Here's how the part is built. I have some questions about the finished solid (model axes, mm). A direction names the side the tool comes from. Coordinates: 2 decimals unless noted, no trailing zeros. Write each loop counter-clockwise with the first axis right and the second up, starting at its lowest first coordinate (ties: lowest second). Pieces come first, ordered by that corner, then holes. Notation, with made-up numbers: (-14, 13) -> (22, 13) arc R33 ccw to (22, 41) -> close; hole circle Ø2 at (68, -35). An arc over 180 degrees is marked (long way). Use a Markdown table: item, result. Add a question column.
Item 1: If I drill on line 1 along Y through (x, z) = (0, -0.5); line 2 along Y through (x, z) = (0, 1.5); line 3 along X through (y, z) = (17.5, -0.5), over which ranges is the centre line in solid material (lowest first)? Write a range as from..to.
Item 2: On a 3-axis mill with a long thin cutter (end or side, diameter ignored), from which of +Z, -Z, +X, -X, +Y, -Y can I reach the whole of each face in a straight line? I mean faces 1 (the cylindrical face through (61.522, 19.374, 0.986)), 2 (the flat face through (22.5, 1, -7)), 3 (the cylindrical face through (-62.44, 2.75, 6.44)), 4 (the flat face through (0, -37.5, -4)), 5 (the flat face through (-22.5, 1, -7)). Say none if no direction works.
Item 3: If we mould it in two halves opening along Y, with no side actions, what happens to faces 6 (the flat face through (0, 37.5, -4)), 7 (the cylindrical face through (-0.54, 19.94, 2.83)), 8 (the flat face through (-34, 53, 2))? For each: pulls with the +Y half, pulls with the -Y half, needs draft (parallel to the pull), parting line crosses it, or undercut.
Item 4: Will these pins go through, and if not, where does the flat tip stop? pin 1 Ø4 at (y, z) = (-29, -4.5) entering from -X; pin 2 Ø8 at (x, y) = (0, 17.5) entering from -Z; pin 3 Ø4.5 at (x, z) = (0, -5.5) entering from -Y.
Item 5: Imagine slicing it at C-C, the plane z = -12. Write out the boundary of the cut face in (x, y), and give its area (3 significant figures).
Item 6: Imagine slicing it at A-A, the plane x = 0. Write out the boundary of the cut face in (y, z).
Item 7: Imagine slicing it at B-B, the plane y = -17.5. Write out the boundary of the cut face in (x, z), and give its area (3 significant figures).
Item 8: Imagine slicing it at D-D, the plane x = -19.5. Write out the boundary of the cut face in (y, z), and give its area (3 significant figures).
```python
from build123d import *

# Parameters (mm, degrees)
F0_R      = 64.5
F1_DEPTH  = 2
F2_R      = 62.5
F3_DEPTH  = 9
F4_W      = 45
F4_H      = 75
F5_DEPTH  = 15
F8_DEPTH  = 75
F9_R      = 2.5
F10_DEPTH = 35


with BuildPart() as f1:
    # F0 (on Top) → F1 (new body)
    with BuildSketch(Plane.XY):
        Circle(F0_R)
    extrude(amount=F1_DEPTH)

    # F2 (on face) → F3 (join)
    with BuildSketch(Plane.XY.offset(2)):
        Circle(F2_R)
    extrude(amount=F3_DEPTH)

    # F4 (on face) → F5 (join)
    with BuildSketch(Plane(origin=(0, 0, 0), x_dir=(1, 0, 0), z_dir=(0, 0, -1))):
        Rectangle(F4_W, F4_H)
    extrude(amount=F5_DEPTH)

    # F7 (on face) → F8 (cut)
    with BuildSketch(Plane.XZ.offset(37.5)):
        with BuildLine():
            Line((-22.360679775, -15), (22.360679775, -15))
            ThreePointArc((22.360679775, -15), (0, -5), (-22.360679775, -15))
        make_face()
    extrude(amount=-F8_DEPTH, mode=Mode.SUBTRACT)

    # F9 (on face) → F10 (cut)
    with BuildSketch(Plane(origin=(0, 0, -15), x_dir=(1, 0, 0), z_dir=(0, 0, -1))):
        with Locations((0, 17.5)):
            Circle(F9_R)
        with Locations((0, -17.5)):
            Circle(F9_R)
    extrude(amount=-F10_DEPTH, mode=Mode.SUBTRACT)


solid = f1.part
```
Ans:
| question | item | result |
|---|---|---|
| 1 | line 1 | y = -37.5..-20, -15..15, 20..37.5 |
| 1 | line 2 | y = -64.5..-20, -15..15, 20..64.5 |
| 1 | line 3 | x = -22.5..-2.5, 2.5..22.5 |
| 2 | face 1 | +Z, -Z |
| 2 | face 2 | -Z, +X, +Y, -Y |
| 2 | face 3 | +Z |
| 2 | face 4 | -Z, +X, -X, -Y |
| 2 | face 5 | -Z, -X, +Y, -Y |
| 3 | face 6 | pulls with the +Y half |
| 3 | face 7 | undercut |
| 3 | face 8 | needs draft |
| 4 | pin 1 | stops at x = -22.5 |
| 4 | pin 2 | stops at z = -5.27 |
| 4 | pin 3 | stops at y = -37.5 |
| 5 | outline | (-22.5, -37.5) -> (-19.26, -37.5) -> (-19.26, 37.5) -> (-22.5, 37.5) -> close; (19.26, -37.5) -> (22.5, -37.5) -> (22.5, 37.5) -> (19.26, 37.5) -> close |
| 5 | area | 486 mm^2 |
| 6 | outline | (-64.5, 0) -> (-37.5, 0) -> (-37.5, -5) -> (-20, -5) -> (-20, 11) -> (-62.5, 11) -> (-62.5, 2) -> (-64.5, 2) -> close; (-15, -5) -> (15, -5) -> (15, 11) -> (-15, 11) -> close; (20, -5) -> (37.5, -5) -> (37.5, 0) -> (64.5, 0) -> (64.5, 2) -> (62.5, 2) -> (62.5, 11) -> (20, 11) -> close |
| 7 | outline | (-62.08, 0) -> (-22.5, 0) -> (-22.5, -15) -> (-22.36, -15) arc R30 cw to (-2.5, -5.1) -> (-2.5, 11) -> (-60, 11) -> (-60, 2) -> (-62.08, 2) -> close; (2.5, -5.1) arc R30 cw to (22.36, -15) -> (22.5, -15) -> (22.5, 0) -> (62.08, 0) -> (62.08, 2) -> (60, 2) -> (60, 11) -> (2.5, 11) -> close |
| 7 | area | 1,610 mm^2 |
| 8 | outline | (-61.48, 0) -> (-37.5, 0) -> (-37.5, -12.2) -> (37.5, -12.2) -> (37.5, 0) -> (61.48, 0) -> (61.48, 2) -> (59.38, 2) -> (59.38, 11) -> (-59.38, 11) -> (-59.38, 2) -> (-61.48, 2) -> close |
| 8 | area | 2,230 mm^2 |
